Geometry: final body of the model. Coordinates: model frame, mm. Face numbers are marked on the shaded views. Give positions to 0.01 mm unless a question says otherwise; leave off trailing zeros. Write each loop counter-clockwise with the first axis right and the second up, starting at its lowest first coordinate (ties: lowest second). Pieces come first, ordered by that corner, then holes.
Q1. Pin query (flat end, axial travel): pin 1 (1.5 mm diameter, centred on x = 0.5, z = 10.5, fed in from -Y); pin 2 (1.5 mm diameter, centred on y = 0.5, z = 3.5, fed in from -X); pin 3 (1.5 mm diameter, centred on x = -1, y = -1, fed in from -Z). Return the tip coordinate at first contact, or that it passes through.
Q2. Draft query along Z for the marked faces 1 and 2. Return one class per face: pulls with the +Z half, pulls with the -Z half, needs draft (parallel to the pull), parting line crosses it, or undercut.
Q3. Cut plane A-A on z = 17. Return the cut outline in (x, y).
Q4. Line query: L1, parallel to Z at x = 1.15, y = -0.85; L2, parallel to Z at x = -1.8, y = -0.4; L3, parallel to Y at x = 0, z = 3.5. Output: solid intervals per line, ascending.
Autodesk Inventor part; units mm, degrees
ref_plane "Work Plane1" through (0, 0, 8.75) normal (0, 0, -1) x (-1, 0, 0)
ref_plane "YZ Plane" through (0, 0, 0) normal (1, 0, 0) x (0, 1, 0)
ref_plane "XZ Plane" through (0, 0, 0) normal (0, 1, 0) x (-1, 0, 0)
sketch "Sketch1" plane through (0, 0, 0) normal (0, 0, 1) x (1, 0, 0)
  circle A0 centre (0, 0) radius 1
  dimension "d0" = 2
extrude "Extrusion1" add sketch "Sketch1" along normal blind 17.5
sketch "Sketch2" plane through (0, 0, 17.5) normal (0, 0, 1) x (1, 0, 0)
  circle A0 centre (0, 0) radius 1
  circle A1 centre (0, 0) radius 2
  dimension "d3" = 4
extrude "Extrusion2" add sketch "Sketch2" along normal blind 1 contours A0 | A1
chamfer "Chamfer1" distance 0.7 distance2 1 1 edges at (-2, 0, 18.5) measured on face at (1.9935, -0.1609, 18.1667)
fillet "Fillet1" radius 2.75 1 edges at (-1, 0, 18.5)
ref_plane "Work Plane1" through (0, 0, 8.75) normal (0, 0, -1) x (-1, 0, 0)
mirror "Mirror1" about plane through (0, 0, 8.75) normal (0, 0, -1) of "Extrusion2", "Chamfer1", "Fillet1"
properties part number "02"
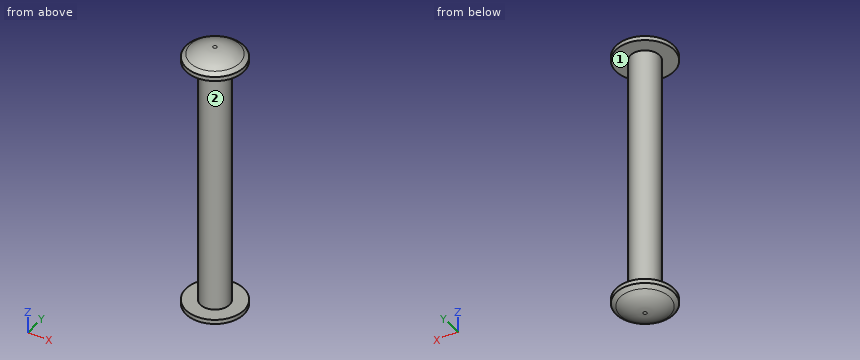
Data:
1. pin 1: stops at y = -1
1. pin 2: stops at x = -1
1. pin 3: stops at z = -0.95
2. face 1: undercut
2. face 2: undercut
3. outline: circle Ø2 at (0, 0)
4. L1: z = -0.67 to 0, 17.5 to 18.17
4. L2: z = -0.41 to 0, 17.5 to 17.91
4. L3: y = -1 to 1
